For this review, use the dimensioned drawing (mm, ordinates from the lowest corner) and the shaded views. A direction names the side the tool comes from. Give positions to 0.01 mm unless a question says otherwise; leave off trailing zeros. Order: outer loops, then holes, each group sorted by start corner. A loop starts at its lowest first (then second) coordinate and runs counter-clockwise, first axis right, second up.
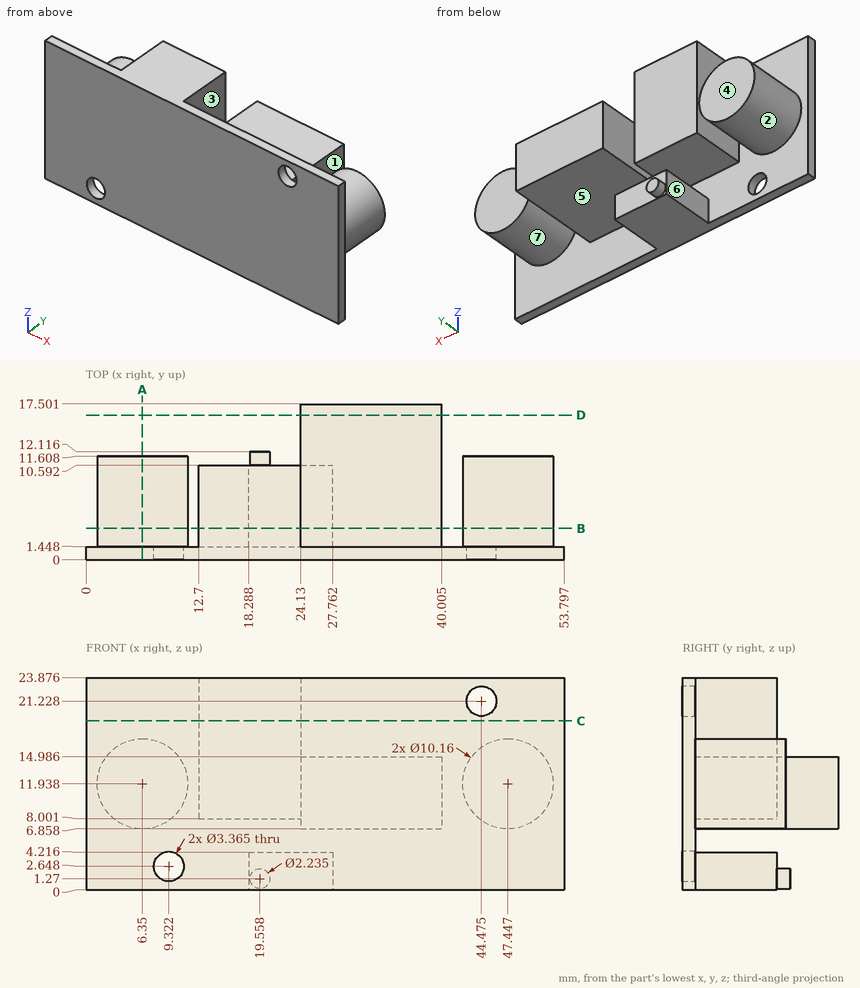
1. Take a section at B-B (y = 3.5). State how many separate pieces and enclosed holes the cut face has.
Recorded:
separate pieces: 4
enclosed holes: 0
2. For pin 1 (4.5 mm diameter, centred on y = 6, z = 3, fed in from -X); pin 2 (6 mm diameter, centred on x = 34.5, y = 6.5, fed in from +Z); pin 3 (4.5 mm diameter, centred on x = 24.5, z = 2, fed in from +Y); pin 4 (2 mm diameter, centred on x = 44.48, z = 21.23, fed in from -Y), all flat-tipped, find the tip position at first contact; note any pin that passes through.
Recorded:
pin 1: stops at x = 18.29
pin 2: stops at z = 14.99
pin 3: stops at y = 10.59
pin 4: passes through
3. Machinability: for the marked faces 1, 2, 3 and 4, which of the approach directions +Z, -Z, +X, -X, +Y, -Y give a long, thin tool a straight path to every point of the face, cutting with its end or side? Answer none if there is none.
Recorded:
face 1: +Z, -Z, +Y
face 2: +Y
face 3: +Z, +Y
face 4: +Z, -Z, -X, +Y
4. For line 1 along X through (y, z) = (2.75, 12) (1 decimal); line 2 along Z through (x, y) = (20, 3.5) (1 decimal); line 3 along X through (y, z) = (7.75, 16.25) (1 decimal), list the stretches that pass through material, from the lowest coordinate up.
Recorded:
line 1: x = 1.3 to 11.4, 12.7 to 40, 42.4 to 52.5
line 2: z = 0 to 4.2, 8 to 23.9
line 3: x = 3.7 to 9, 12.7 to 24.1, 44.8 to 50.1
5. Take a section at C-C (z = 19). State the section outline as (x, y) points.
Recorded:
outline: (0, 0) - (53.8, 0) - (53.8, 1.45) - (24.13, 1.45) - (24.13, 10.59) - (12.7, 10.59) - (12.7, 1.45) - (0, 1.45) - close
6. Take a section at D-D (y = 16.25). State the section outline as (x, z) points (1 decimal).
Recorded:
outline: (24.1, 6.9) - (40, 6.9) - (40, 15) - (24.1, 15) - close
7. Draft analysis for pull direction X (two halves, no side actions). For the marked faces 5, 6 and 7, state which applies: pulls with the +X half, pulls with the -X half, needs draft (parallel to the pull), parting line crosses it, or undercut.
Recorded:
face 5: needs draft
face 6: pulls with the -X half
face 7: undercut
8. Take a section at A-A (x = 6.35). State the section outline as (y, z) points (1 decimal), then the cut area to 3 significant figures.
Recorded:
outline: (0, 0) - (1.4, 0) - (1.4, 6.9) - (11.6, 6.9) - (11.6, 17) - (1.4, 17) - (1.4, 23.9) - (0, 23.9) - close
area: 138 mm2
